Geometry: final body of the model. Coordinates: model frame, mm. A direction names the side the tool comes from. Round coordinates to 2 decimals unless told otherwise and drop trailing zeros. Loops run counter-clockwise (first coordinate to the right, second up) from the corner with the lowest first, then second, coordinate; pieces in that order, holes last. Notation, with made-up numbers: (3.25, 65.25) -> (25.25, 65.25) arc R7 ccw to (25.25, 78.25) -> close; hole circle Ø9 at (57.5, 48). An arc over 180 degrees is marked (long way). Answer in a Markdown table with one row per item.
```python
from build123d import *

# Parameters (mm, degrees)
EXTRUDE_1_DEPTH     = 11.5
CUT_EXTRUDE_1_DEPTH = 11.5
CUT_EXTRUDE_2_DEPTH = 11.5
CUT_EXTRUDE_3_DEPTH = 1.8
CUT_EXTRUDE_4_DEPTH = 1.8
CUT_EXTRUDE_5_DEPTH = 1.8
CUT_EXTRUDE_6_DEPTH = 1.8
FILLET_1_R          = 2
FILLET_2_R          = 2
FILLET_3_R          = 1
FILLET_4_R          = 1


with BuildPart() as part:
    # 草图1 → 凸台-拉伸1 (new body)
    with BuildSketch(Plane.XY):
        Polygon((14.4, 3.2), (14.4, 11.25), (0, 11.25), (0, 3.2), (-5.5, 3.2), (-5.5, 0), (0, 0), (1.3, 0), (1.3, 9.85), (13.1, 9.85), (13.1, 0), (14.4, 0), (19.9, 0), (19.9, 3.2), align=None)
    extrude(amount=EXTRUDE_1_DEPTH)

    # 草图2 → 切除-拉伸1 (cut)
    with BuildSketch(Plane(origin=(0, 3.2, 0), x_dir=(1, 0, 0), z_dir=(0, 1, 0))):
        with BuildLine():
            Line((14.4, 0), (14.4, -3.1))
            Line((14.4, -3.1), (15.7, -3.1))
            ThreePointArc((15.7, -3.1), (18.669848481, -4.330151519), (19.9, -7.3))
            Line((19.9, -7.3), (19.9, 0))
            Line((19.9, 0), (14.4, 0))
        make_face()
        with BuildLine():
            ThreePointArc((19.9, -7.3), (18.669848481, -10.269848481), (15.7, -11.5))
            Line((15.7, -11.5), (19.9, -11.5))
            Line((19.9, -11.5), (19.9, -7.3))
        make_face()
    extrude(amount=-CUT_EXTRUDE_1_DEPTH, mode=Mode.SUBTRACT)

    # 草图3 → 切除-拉伸2 (cut)
    with BuildSketch(Plane(origin=(0, 3.2, 0), x_dir=(1, 0, 0), z_dir=(0, 1, 0))):
        with BuildLine():
            Line((-1.3, -3.1), (0, -3.1))
            Line((0, -3.1), (0, 0))
            Line((0, 0), (-5.5, 0))
            Line((-5.5, 0), (-5.5, -7.3))
            ThreePointArc((-5.5, -7.3), (-4.269848481, -4.330151519), (-1.3, -3.1))
        make_face()
        with BuildLine():
            Line((-5.5, -11.5), (-1.3, -11.5))
            ThreePointArc((-1.3, -11.5), (-4.269848481, -10.269848481), (-5.5, -7.3))
            Line((-5.5, -7.3), (-5.5, -11.5))
        make_face()
    extrude(amount=-CUT_EXTRUDE_2_DEPTH, mode=Mode.SUBTRACT)

    # 草图5 → 切除-拉伸3 (cut)
    with BuildSketch(Plane(origin=(0, 3.2, 0), x_dir=(1, 0, 0), z_dir=(0, 1, 0))):
        Polygon((18.6, -6.087564435), (16.5, -4.875128869), (14.4, -6.087564435), (14.4, -8.512435565), (16.5, -9.724871131), (18.6, -8.512435565), align=None)
    extrude(amount=-CUT_EXTRUDE_3_DEPTH, mode=Mode.SUBTRACT)

    # 草图8 → 切除-拉伸4 (cut)
    with BuildSketch(Plane(origin=(0, 3.2, 0), x_dir=(1, 0, 0), z_dir=(0, 1, 0))):
        Polygon((-4.2, -6.087564435), (-4.2, -8.512435565), (-2.1, -9.724871131), (0, -8.512435565), (0, -6.087564435), (-2.1, -4.875128869), align=None)
    extrude(amount=-CUT_EXTRUDE_4_DEPTH, mode=Mode.SUBTRACT)

    # 草图10 → 切除-拉伸5 (cut)
    with BuildSketch(Plane(origin=(0, 1.4, 0), x_dir=(1, 0, 0), z_dir=(0, 1, 0))):
        with BuildLine():
            Line((0, -8.425), (0, -6.175))
            Line((0, -6.175), (-2.1, -6.175))
            ThreePointArc((-2.1, -6.175), (-3.225, -7.3), (-2.1, -8.425))
            Line((-2.1, -8.425), (0, -8.425))
        make_face()
    extrude(amount=-CUT_EXTRUDE_5_DEPTH, mode=Mode.SUBTRACT)

    # 草图7 → 切除-拉伸6 (cut)
    with BuildSketch(Plane(origin=(0, 1.4, 0), x_dir=(1, 0, 0), z_dir=(0, 1, 0))):
        with BuildLine():
            Line((14.4, -6.175), (14.4, -8.425))
            Line((14.4, -8.425), (16.5, -8.425))
            ThreePointArc((16.5, -8.425), (17.625, -7.3), (16.5, -6.175))
            Line((16.5, -6.175), (14.4, -6.175))
        make_face()
    extrude(amount=-CUT_EXTRUDE_6_DEPTH, mode=Mode.SUBTRACT)

    # 圆角1
    fillet_1_edges = [part.edges().sort_by_distance(p)[0] for p in [
        (0, 11.25, 5.75),
    ]]
    fillet(fillet_1_edges, radius=FILLET_1_R)

    # 圆角2
    fillet_2_edges = [part.edges().sort_by_distance(p)[0] for p in [
        (14.4, 11.25, 5.75),
    ]]
    fillet(fillet_2_edges, radius=FILLET_2_R)

    # 圆角3
    fillet_3_edges = [part.edges().sort_by_distance(p)[0] for p in [
        (1.3, 9.85, 5.75),
    ]]
    fillet(fillet_3_edges, radius=FILLET_3_R)

    # 圆角4
    fillet_4_edges = [part.edges().sort_by_distance(p)[0] for p in [
        (13.1, 9.85, 5.75),
    ]]
    fillet(fillet_4_edges, radius=FILLET_4_R)


solid = part.part
```
Item 1: Set-up query: faces 1 (the flat face through (13.1, 4, 6)), 2 (the flat face through (15, 1, 6.175)), 3 (the flat face through (18, 1.4, 7)), 4 (the flat face through (7, 10, 0)). Return all of +Z, -Z, +X, -X, +Y, -Y with unobstructed straight access to the full face (end or side cutting, diameter ignored); none if empty.
Ans:
| item | result |
|---|---|
| face 1 | +Z, -Z, -Y |
| face 2 | +Y, -Y |
| face 3 | +Y |
| face 4 | -Z, +X, -X, +Y, -Y |
Item 2: Section query A-A, the plane y = 5.5. Output: boundary loops of the cut face in (x, z).
Ans:
| item | result |
|---|---|
| outline | (0, 0) -> (1.3, 0) -> (1.3, 11.5) -> (0, 11.5) -> close; (13.1, 0) -> (14.4, 0) -> (14.4, 11.5) -> (13.1, 11.5) -> close |
Item 3: Mould query, pull axis Z, two halves, no side actions, for faces 5 (the flat face through (-4.2, 2, 7)), 6 (the flat face through (18, 3.2, 5)), 7 (the flat face through (7, 10, 11.5)). Classes: released by +Z, released by -Z, zero draft, split by the parting line, or undercut.
Ans:
| item | result |
|---|---|
| face 5 | undercut |
| face 6 | zero draft |
| face 7 | released by +Z |
Item 4: Ray query, L1, parallel to X at y = 5.25, z = 0.5; L2, parallel to Z at x = -0.25, y = 1.25 (3 decimals); L3, parallel to Y at x = 6.75, z = 10.75. Return the intervals inside material, ascending.
Ans:
| item | result |
|---|---|
| L1 | 0 to 1.3, 13.1 to 14.4 |
| L2 | 3.1 to 6.175, 8.425 to 11.5 |
| L3 | 9.85 to 11.25 |
Item 5: Section query C-C, the plane x = 17. Output: boundary loops of the cut face in (y, z).
Ans:
| item | result |
|---|---|
| outline | (0, 3.31) -> (3.2, 3.31) -> (3.2, 5.16) -> (1.4, 5.16) -> (1.4, 6.29) -> (0, 6.29) -> close; (0, 8.31) -> (1.4, 8.31) -> (1.4, 9.44) -> (3.2, 9.44) -> (3.2, 11.29) -> (0, 11.29) -> close |
Item 6: Section query D-D, the plane x = -3.5. Output: boundary loops of the cut face in (y, z), and give its area (3 significant figures).
Ans:
| item | result |
|---|---|
| outline | (0, 3.72) -> (3.2, 3.72) -> (3.2, 5.68) -> (1.4, 5.68) -> (1.4, 8.92) -> (3.2, 8.92) -> (3.2, 10.88) -> (0, 10.88) -> close |
| area | 17.1 mm2 |
Item 7: Section query B-B, the plane z = 2.75. Output: boundary loops of the cut face in (x, y), and give its area (3 significant figures).
Ans:
| item | result |
|---|---|
| outline | (0, 0) -> (1.3, 0) -> (1.3, 8.85) arc R1 cw to (2.3, 9.85) -> (12.1, 9.85) arc R1 cw to (13.1, 8.85) -> (13.1, 0) -> (14.4, 0) -> (14.4, 9.25) arc R2 ccw to (12.4, 11.25) -> (2, 11.25) arc R2 ccw to (0, 9.25) -> close |
| area | 44.5 mm2 |
Item 8: First-contact query: P1, Ø2, axis at y = 5, z = 8.5, coming from the -X side; P2, Ø1, axis at x = 16, z = 7, coming from the +Y side; P3, Ø4.5, axis at x = -1.5, z = 9.5, coming from the +Y side; P4, Ø0.7, axis at x = 15, y = 1, coming from the -Z side. Flat tips, straight axial feed; report the tip coordinate or a pass-through.
Ans:
| item | result |
|---|---|
| P1 | x = 0 |
| P2 | through |
| P3 | y = 10.81 |
| P4 | z = 3.1 |
